from build123d import *

# Parameters (mm, degrees)
SKETCH_1_W                   = 37
SKETCH_1_H                   = 30
SKETCH_1_R                   = 12.5
EXTRUDE_1_DEPTH              = 5.5
HOLE_WIZARD_M3_1_D           = 2.5
HOLE_WIZARD_M3_1_CSINK_D     = 3.05
HOLE_WIZARD_M3_1_CSINK_ANGLE = 90


with BuildPart() as part:
    # 草图1 → 凸台-拉伸1 (new body)
    with BuildSketch(Plane.XY):
        Rectangle(SKETCH_1_W, SKETCH_1_H)
        Circle(SKETCH_1_R, mode=Mode.SUBTRACT)
    extrude(amount=EXTRUDE_1_DEPTH)

    # M3 螺纹孔1 (through all)
    with Locations(Plane(origin=(0, 15, 0), x_dir=(1, 0, 0), z_dir=(0, 1, 0))):
        with Locations((-15.5, -2.75), (15.5, -2.75)):
            CounterSinkHole(HOLE_WIZARD_M3_1_D / 2, HOLE_WIZARD_M3_1_CSINK_D / 2, counter_sink_angle=HOLE_WIZARD_M3_1_CSINK_ANGLE)


solid = part.part
Work out the finished part from the listing and answer in its coordinate system (mm). Give positions to 0.01 mm unless a question says otherwise; leave off trailing zeros. Order: outer loops, then holes, each group sorted by start corner. A loop starts at its lowest first (then second) coordinate and runs counter-clockwise, first axis right, second up. Notation, with made-up numbers: (41, 3.25) -> (90, 3.25) arc R24 ccw to (90, 28.25) -> close; hole circle Ø9 at (76, 29). An arc over 180 degrees is marked (long way). Answer as a JSON object with one key per item and string values. Group by question number.
1. Section A-A on y = 0 is taken. Determine the outline of the cut face in (x, z), plus the area to 3 significant figures.
2. Section C-C on x = -7.5 is taken. Determine the outline of the cut face in (y, z).
3. Consider line 1 along Z through (x, y) = (15.5, 8); line 2 along Y through (x, z) = (0, 1.3); line 3 along X through (y, z) = (-6.5, 2.4). Determine where each line is inside the solid, lowest interval first. Write a range as [from, to].
4. The mould has two halves that part along X. Classify faces 1 (the cylindrical face through (16.75, -0.35, 2.7)), 2 (the cylindrical face through (-14.579, -0.346, 1.905)), 3 (the flat face through (0, -15, 3)), 4 (the flat face through (18.5, 0, 3)): released by +X, released by -X, zero draft, split by the parting line, or undercut.
5. Section D-D on y = 8.75 is taken. Determine the outline of the cut face in (x, z).
6. A flat-ended cylindrical pin translates along its axis: pin 1 Ø3 at (x, z) = (-15.5, 2.75) entering from +Y (3 decimals). Find the tip coordinate at first contact, or state that the pin passes through.
7. Section B-B on z = 2.75 is taken. Determine the outline of the cut face in (x, y) (3 decimals), plus the area to 3 significant figures.
Result sheet:
{
 "1": {"outline": "(-18.5, 0) -> (-12.5, 0) -> (-12.5, 5.5) -> (-18.5, 5.5) -> close; (12.5, 0) -> (18.5, 0) -> (18.5, 5.5) -> (12.5, 5.5) -> close; hole circle Ø2.5 at (-15.5, 2.75); hole circle Ø2.5 at (15.5, 2.75)", "area": "56.2 mm^2"},
 "2": {"outline": "(-15, 0) -> (-10, 0) -> (-10, 5.5) -> (-15, 5.5) -> close; (10, 0) -> (15, 0) -> (15, 5.5) -> (10, 5.5) -> close"},
 "3": {"line 1": "z = [0, 1.5], [4, 5.5]", "line 2": "y = [-15, -12.5], [12.5, 15]", "line 3": "x = [-18.5, -16.7], [-14.3, -10.68], [10.68, 14.3], [16.7, 18.5]"},
 "4": {"face 1": "undercut", "face 2": "undercut", "face 3": "zero draft", "face 4": "released by +X"},
 "5": {"outline": "(-18.5, 0) -> (-8.93, 0) -> (-8.93, 5.5) -> (-18.5, 5.5) -> close; (8.93, 0) -> (18.5, 0) -> (18.5, 5.5) -> (8.93, 5.5) -> close; hole circle Ø2.5 at (-15.5, 2.75); hole circle Ø2.5 at (15.5, 2.75)"},
 "6": {"pin 1": "stops at y = 14.975"},
 "7": {"outline": "(-18.5, -15) -> (-16.75, -15) -> (-16.75, 14.725) -> (-17.025, 15) -> (-18.5, 15) -> close; (-14.25, -15) -> (14.25, -15) -> (14.25, 14.725) -> (13.975, 15) -> (-13.975, 15) -> (-14.25, 14.725) -> close; (16.75, -15) -> (18.5, -15) -> (18.5, 15) -> (17.025, 15) -> (16.75, 14.725) -> close; hole circle Ø25 at (0, 0)", "area": "469 mm^2"}
}
